Geometry check sheet. Reference: the model listing, model coordinates, mm. A direction names the side the tool comes from. Give positions to 0.01 mm unless a question says otherwise; leave off trailing zeros. Order: outer loops, then holes, each group sorted by start corner. A loop starts at its lowest first (then second) coordinate and runs counter-clockwise, first axis right, second up. Notation, with made-up numbers: M 80,-10 L 134,-10 A17 cw 134,16 Z; hole C 72.5,-16 d1. An arc over 180 degrees is marked long. Answer as CSV lines item,"result". Start each with the question number.
```python
from build123d import *

# Parameters (mm, degrees)
BOSS_EXTRUDE5_START             = -19
BOSS_EXTRUDE5_DEPTH             = 38
CUT_EXTRUDE1_START              = -2.4
CUT_EXTRUDE1_DEPTH              = 2.4
BOSS_EXTRUDE4_REACH             = 47.398
SKETCH5_R                       = 2.6
BOSS_EXTRUDE4_DIRECTION_2_REACH = 47.398
CUT_EXTRUDE3_DEPTH              = 48.70492637
CUT_EXTRUDE3_DEPTH_BACK         = 48.70492637
FILLET17_R                      = 0.4
FILLET_1_R                      = 2.5
HOLE_WIZARD_M41_D               = 4.2
HOLE_WIZARD_M41_DEPTH           = 8.5
HOLE_WIZARD_M41_CSINK_D         = 9.4
HOLE_WIZARD_M41_CSINK_ANGLE     = 90
HOLE_WIZARD_M41_TIP             = 1.2618073


# Read off the part's stored shape, not the designer's step: Boss-Extrude5
with BuildPart() as part:
    # Boss-Extrude5 outline → Boss-Extrude5 (new body)
    with BuildSketch(Plane(origin=(0, 0, 0), x_dir=(0, 0, -1), z_dir=(1, 0, 0)).offset(BOSS_EXTRUDE5_START)):
        with BuildLine():
            Line((0, -10), (40, -10))
            Line((40, -10), (40, 0))
            Line((40, 0), (36.020092303, 9.608347138))
            ThreePointArc((36.020092303, 9.608347138), (31.951342699, 6.586282384), (29.794119342, 2))
            Line((29.794119342, 2), (0, 2))
            Line((0, 2), (0, -10))
        make_face()
    extrude(amount=BOSS_EXTRUDE5_DEPTH)

    # Sketch4 → Cut-Extrude1 (cut)
    with BuildSketch(Plane(origin=(19, 0, 0), x_dir=(0, 0, -1), z_dir=(1, 0, 0)).offset(CUT_EXTRUDE1_START)):
        with BuildLine():
            Line((32.646089476, 7.353910524), (50.4, 25.107821049))
            Line((50.4, 25.107821049), (50.4, 0))
            ThreePointArc((50.4, 0), (36.020092303, -9.608347138), (32.646089476, 7.353910524))
        make_face()
    cut_extrude1 = extrude(amount=CUT_EXTRUDE1_DEPTH, mode=Mode.SUBTRACT)

    # Mirror1: Cut-Extrude1 across plane
    add(cut_extrude1.mirror(Plane(origin=(0, 0, 0), x_dir=(0, 0, 1), z_dir=(1, 0, 0))), mode=Mode.SUBTRACT)

    # Boss-Extrude4: up to this face of the body (flat: up to its plane)
    boss_extrude4_end = Plane(part.part.faces().sort_by_distance((19, -4.194169539, -15.691958581))[0])
    # Sketch5 → Boss-Extrude4 (add, up to the picked face)
    with BuildSketch(Plane(origin=(0, 0, 0), x_dir=(0, 0, -1), z_dir=(1, 0, 0)), mode=Mode.PRIVATE) as boss_extrude4_sk1:
        with Locations((40, 0)):
            Circle(SKETCH5_R)
    boss_extrude4_tool1 = split(extrude(boss_extrude4_sk1.sketch, amount=BOSS_EXTRUDE4_REACH, mode=Mode.PRIVATE), bisect_by=boss_extrude4_end, keep=Keep.BOTH, mode=Mode.PRIVATE)
    add(boss_extrude4_tool1.solids().sort_by(Axis((0, 0, -40), (1, 0, 0)))[0])

    # Boss-Extrude4 direction 2: up to this face of the body (flat: up to its plane)
    boss_extrude4_direction_2_end = Plane(part.part.faces().sort_by_distance((-19, -4.194169539, -15.691958581))[0])
    # Sketch5 → Boss-Extrude4 direction 2 (add, up to the picked face)
    with BuildSketch(Plane(origin=(0, 0, 0), x_dir=(0, 0, -1), z_dir=(1, 0, 0)), mode=Mode.PRIVATE) as boss_extrude4_direction_2_sk1:
        with Locations((40, 0)):
            Circle(SKETCH5_R)
    boss_extrude4_direction_2_tool1 = split(extrude(boss_extrude4_direction_2_sk1.sketch, amount=-BOSS_EXTRUDE4_DIRECTION_2_REACH, mode=Mode.PRIVATE), bisect_by=boss_extrude4_direction_2_end, keep=Keep.BOTH, mode=Mode.PRIVATE)
    add(boss_extrude4_direction_2_tool1.solids().sort_by(Axis((0, 0, -40), (-1, 0, 0)))[0])

    # Sketch7 → Cut-Extrude3 (cut, two sides: drawn at the far end of the back side and taken through both)
    with BuildSketch(Plane.XY.offset(-CUT_EXTRUDE3_DEPTH_BACK)):
        with BuildLine():
            Line((-14.8, -7.5), (14.8, -7.5))
            ThreePointArc((14.8, -7.5), (14.941421356, -7.441421356), (15, -7.3))
            Line((15, -7.3), (15, 12.3))
            ThreePointArc((15, 12.3), (14.941421356, 12.441421356), (14.8, 12.5))
            Line((14.8, 12.5), (-14.8, 12.5))
            ThreePointArc((-14.8, 12.5), (-14.941421356, 12.441421356), (-15, 12.3))
            Line((-15, 12.3), (-15, -7.3))
            ThreePointArc((-15, -7.3), (-14.941421356, -7.441421356), (-14.8, -7.5))
        make_face()
    extrude(amount=CUT_EXTRUDE3_DEPTH + CUT_EXTRUDE3_DEPTH_BACK, mode=Mode.SUBTRACT)

    # Fillet17
    fillet17_edges = [part.edges().sort_by_distance(p)[0] for p in [
        (-19, 0, -37.4),
        (19, 0, -37.4),
        (-16.6, -0.507234837, -37.449958271),
        (16.6, -0.507234837, -37.449958271),
        (16.6, -5.431674396, -31.13112672),
        (-16.6, -5.431674396, -31.13112672),
    ]]
    fillet(fillet17_edges, radius=FILLET17_R)

    # Скругление1
    fillet_1_edges = [part.edges().sort_by_distance(p)[0] for p in [
        (17, 2, 0),
        (-17, 2, 0),
    ]]
    fillet(fillet_1_edges, radius=FILLET_1_R)

    # Зенковка для винта с полупотайной головкой M41
    with Locations(Plane(origin=(-9, -7.5, -8), x_dir=(0, 0, 1), z_dir=(0, 1, 0))):
        with Locations((0, 0), (0, 18)):
            CounterSinkHole(HOLE_WIZARD_M41_D / 2, HOLE_WIZARD_M41_CSINK_D / 2, depth=HOLE_WIZARD_M41_DEPTH, counter_sink_angle=HOLE_WIZARD_M41_CSINK_ANGLE)
            with Locations((0, 0, -(HOLE_WIZARD_M41_DEPTH + HOLE_WIZARD_M41_TIP / 2))):  # 118° drill point
                Cone(0, HOLE_WIZARD_M41_D / 2, HOLE_WIZARD_M41_TIP, mode=Mode.SUBTRACT)


solid = part.part
```
Item 1: Section check D-D on z = -25. Record the boundary of the cut face in (x, y).
Item 2: Scan lines: line 1 along X through (y, z) = (7, -34.5); line 2 along X through (y, z) = (1.25, -16); line 3 along Y through (x, z) = (8, -21.5). Record each from-to range of solid material in increasing order.
Item 3: Access from +Z, -Z, +X, -X, +Y, -Y to the whole of each face (thin tool, end or side, straight path). Record for faces 1 (the face through (17.028, 1.248, -0.713)), 2 (the face through (-16.6, 0, -35)), 3 (the face through (15, -1, -22)).
Item 4: Section check B-B on z = -8. Record the boundary of the cut face in (x, y).
Item 5: Section check C-C on y = 6. Record the boundary of the cut face in (x, z).
Item 6: Section check A-A on x = 9. Record the boundary of the cut face in (y, z), then the cut area to 4 significant figures.
Item 7: Draft check along Z on faces 4 (the face through (17.17, 0.78, -42.48)), 5 (the face through (-19, 0, -40)), 6 (the face through (-16.972, 1.287, -0.752)). Enter one of: pulls with the +Z half, pulls with the -Z half, needs draft (parallel to the pull), parting line crosses it, or undercut.
Item 8: Depth check by flat-ended pin: pin 1 Ø4.5 at (x, z) = (-16.5, -13.5) entering from +Y; pin 2 Ø10 at (x, z) = (8, -9) entering from +Y; pin 3 Ø3 at (x, z) = (7.5, -8.5) entering from +Y. Enter the tip coordinate at first touch or a pass-through.
Numbers:
1,outline,"M -19,-10 L 19,-10 L 19,2 L 15,2 L 15,-7.3 A0.2 cw 14.8,-7.5 L -14.8,-7.5 A0.2 cw -15,-7.3 L -15,2 L -19,2 Z"
2,line 1,"-16.6 to -15, 15 to 16.6"
2,line 2,"-19 to -15, 15 to 19"
2,line 3,"-10 to -7.5"
3,face 1,"+Z, +X, -X, +Y"
3,face 2,"-X"
3,face 3,"+Z, -Z, +Y"
4,outline,"M -19,-10 L -11.2,-10 L -13.7,-7.5 L -14.8,-7.5 A0.2 cw -15,-7.3 L -15,2 L -19,2 Z; M -6.8,-10 L 6.8,-10 L 4.3,-7.5 L -4.3,-7.5 Z; M 11.2,-10 L 19,-10 L 19,2 L 15,2 L 15,-7.3 A0.2 cw 14.8,-7.5 L 13.7,-7.5 Z"
5,outline,"M -16.6,-37.51 L -15,-37.51 L -15,-31.51 L -16.6,-31.51 Z; M 15,-37.51 L 16.6,-37.51 L 16.6,-31.51 L 15,-31.51 Z"
6,outline,"M -10,-40 L -7.5,-40 L -7.5,-12.7 L -10,-10.2 Z; M -10,-5.8 L -7.5,-3.3 L -7.5,0 L -10,0 Z"
6,area,"82.75 mm2"
7,face 4,"undercut"
7,face 5,"needs draft"
7,face 6,"pulls with the +Z half"
8,pin 1,"y = 2"
8,pin 2,"y = -7.5"
8,pin 3,"y = -9.12"
